```python
from build123d import *

# Parameters (mm, degrees)
BOSS_EXTRUDE1_DEPTH = 5


with BuildPart() as part:
    # Sketch1 → Boss-Extrude1 (new body)
    with BuildSketch(Plane.XY):
        with BuildLine():
            Line((-114.983429669, -41.595326503), (-88.552733296, -41.595326503))
            ThreePointArc((-88.552733296, -41.595326503), (-84.32255291, -43.929698265), (-80.092372525, -41.595326503))
            Line((-80.092372525, -41.595326503), (-58.788151834, -41.595326503))
            Line((-58.788151834, -41.595326503), (-42.04280008, -12.591526475))
            ThreePointArc((-42.04280008, -12.591526475), (-39.562725839, -10.795911883), (-39.247715108, -7.750297292))
            Line((-39.247715108, -7.750297292), (-24.147135682, 18.404673497))
            Line((-24.147135682, 18.404673497), (49.753698774, 18.404673497))
            Line((49.753698774, 18.404673497), (64.843098402, -7.730933315))
            ThreePointArc((64.843098402, -7.730933315), (65.07717154, -10.998946288), (67.790317225, -12.835666057))
            Line((67.790317225, -12.835666057), (84.394714925, -41.595326503))
            Line((84.394714925, -41.595326503), (105.408163945, -41.595326503))
            ThreePointArc((105.408163945, -41.595326503), (109.928281546, -44.457912909), (114.448399147, -41.595326503))
            Line((114.448399147, -41.595326503), (140.300890001, -41.595326503))
            ThreePointArc((140.300890001, -41.595326503), (144.821007602, -44.457912909), (149.341125203, -41.595326503))
            Line((149.341125203, -41.595326503), (170.354574223, -41.595326503))
            Line((170.354574223, -41.595326503), (170.354574223, 149.258117984))
            Line((170.354574223, 149.258117984), (94.234420776, 149.258117984))
            ThreePointArc((94.234420776, 149.258117984), (89.904293757, 151.758117984), (85.574166738, 149.258117984))
            Line((85.574166738, 149.258117984), (-59.967510158, 149.258117984))
            ThreePointArc((-59.967510158, 149.258117984), (-64.297637177, 151.758117984), (-68.627764196, 149.258117984))
            Line((-68.627764196, 149.258117984), (-144.748011131, 149.258117984))
            Line((-144.748011131, 149.258117984), (-144.748011131, -41.595326503))
            Line((-144.748011131, -41.595326503), (-123.44379044, -41.595326503))
            ThreePointArc((-123.44379044, -41.595326503), (-119.213610054, -43.929698265), (-114.983429669, -41.595326503))
        make_face()
    extrude(amount=BOSS_EXTRUDE1_DEPTH)


solid = part.part
```
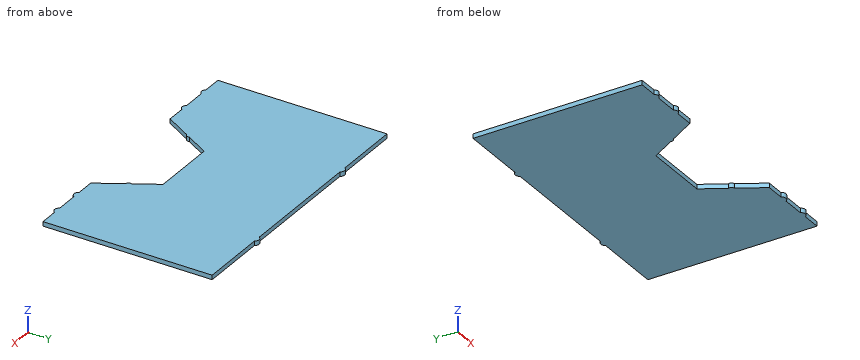
Read the model definition and answer for the solid it produces. Units are mm, in the model's axes. Coordinates: 2 decimals unless noted, no trailing zeros. Write each loop counter-clockwise with the first axis right and the second up, starting at its lowest first coordinate (ties: lowest second). Pieces come first, ordered by that corner, then holes. Notation, with made-up numbers: (-34, -24.5) -> (23, -24.5) arc R21 ccw to (23, 4.5) -> close; hole circle Ø5 at (88.5, 33). An arc over 180 degrees is marked (long way). Return JSON: item names as keys, results as strings.
1. A cutting plane is placed at D-D (x = 12). Determine the outline of the cut face in (y, z).
Found:
{"outline": "(18.4, 0) -> (149.26, 0) -> (149.26, 5) -> (18.4, 5) -> close"}
2. A cutting plane is placed at C-C (x = 133.5). Determine the outline of the cut face in (y, z), and give its area (3 significant figures).
Found:
{"outline": "(-41.6, 0) -> (149.26, 0) -> (149.26, 5) -> (-41.6, 5) -> close", "area": "954 mm2"}
3. A cutting plane is placed at A-A (z = 3.55). Determine the outline of the cut face in (x, y).
Found:
{"outline": "(-144.75, -41.6) -> (-123.44, -41.6) arc R5 ccw to (-114.98, -41.6) -> (-88.55, -41.6) arc R5 ccw to (-80.09, -41.6) -> (-58.79, -41.6) -> (-42.04, -12.59) arc R3.75 ccw to (-39.25, -7.75) -> (-24.15, 18.4) -> (49.75, 18.4) -> (64.84, -7.73) arc R3.75 ccw to (67.79, -12.84) -> (84.39, -41.6) -> (105.41, -41.6) arc R5 ccw to (114.45, -41.6) -> (140.3, -41.6) arc R5 ccw to (149.34, -41.6) -> (170.35, -41.6) -> (170.35, 149.26) -> (94.23, 149.26) arc R5 ccw to (85.57, 149.26) -> (-59.97, 149.26) arc R5 ccw to (-68.63, 149.26) -> (-144.75, 149.26) -> close"}
4. Each of these flat-tipped pins is pushed along its axis until it touches: P1, Ø2.5, axis at x = 129.5, z = 3, coming from the -Y side; P2, Ø1.5, axis at x = 8, z = 2, coming from the -Y side; P3, Ø2.5, axis at x = 7.5, z = 1.5, coming from the +Y side. Where does it stop, or does it pass through?
Found:
{"P1": "y = -41.6", "P2": "y = 18.4", "P3": "y = 149.26"}
5. Find the intervals of material crossed by line 1 along Y through (x, z) = (-111, 4.7); line 2 along Y through (x, z) = (-8, 3.55); line 3 along X through (y, z) = (-1, 2.55), in increasing order. Write a range as from..to.
Found:
{"line 1": "-41.6..149.26", "line 2": "18.4..149.26", "line 3": "-144.75..-35.35, 60.96..170.35"}
6. A cutting plane is placed at B-B (y = -20.5). Determine the outline of the cut face in (x, z).
Found:
{"outline": "(-144.75, 0) -> (-46.61, 0) -> (-46.61, 5) -> (-144.75, 5) -> close; (72.22, 0) -> (170.35, 0) -> (170.35, 5) -> (72.22, 5) -> close"}
